Read the model definition and answer for the solid it produces. Units are mm, in the model's axes. A direction names the side the tool comes from. Coordinates: 2 decimals unless noted, no trailing zeros. Order: outer loops, then holes, each group sorted by start corner. A loop starts at its lowest first (then second) coordinate and runs counter-clockwise, first axis right, second up. Notation, with made-up numbers: (63.25, 60) -> (108.25, 60) arc R5 ccw to (108.25, 69) -> close; hole circle Ø6 at (-37.5, 23). An arc over 180 degrees is marked (long way). Answer in a Markdown table with one row per item.
from build123d import *

# Parameters (mm, degrees)
SKETCH1_W           = 73
SKETCH1_H           = 4
BOSS_EXTRUDE1_DEPTH = 200
SKETCH2_R           = 1.5
SKETCH2_W           = 40.5
SKETCH2_H           = 21
CUT_EXTRUDE1_DEPTH  = 2000


with BuildPart() as part:
    # Sketch1 → Boss-Extrude1 (new body)
    with BuildSketch(Plane(origin=(0, 0, 0), x_dir=(0, 0, -1), z_dir=(1, 0, 0))):
        Rectangle(SKETCH1_W, SKETCH1_H)
    extrude(amount=-BOSS_EXTRUDE1_DEPTH)

    # Sketch2 → Cut-Extrude1 (cut)
    with BuildSketch(Plane(origin=(0, 2, 0), x_dir=(1, 0, 0), z_dir=(0, 1, 0))):
        with Locations(Location((-186, 1.5, 0), (0, 0, 270))):
            Circle(SKETCH2_R)
        with Locations(Location((-133.5, 1.5, 0), (0, 0, 90))):
            Circle(SKETCH2_R)
        with Locations((-159.75, 1.5)):
            Rectangle(SKETCH2_W, SKETCH2_H)
    extrude(amount=-CUT_EXTRUDE1_DEPTH, mode=Mode.SUBTRACT)


solid = part.part
Q1. The part is cut by section A-A (x = -146). Write down the section's boundary in (y, z), then the cut area to 3 significant figures.
Outcome:
| item | result |
|---|---|
| outline | (-2, -36.5) -> (2, -36.5) -> (2, -12) -> (-2, -12) -> close; (-2, 9) -> (2, 9) -> (2, 36.5) -> (-2, 36.5) -> close |
| area | 208 mm² |
Q2. The part is cut by section B-B (y = -0.8). Write down the section's boundary in (x, z).
Outcome:
| item | result |
|---|---|
| outline | (-200, -36.5) -> (0, -36.5) -> (0, 36.5) -> (-200, 36.5) -> close; hole circle Ø3 at (-186, -1.5); hole (-180, -12) -> (-139.5, -12) -> (-139.5, 9) -> (-180, 9) -> close; hole circle Ø3 at (-133.5, -1.5) |
Q3. For faces 4 (the face through (-99, 0, -36.5)), 5 (the face through (-160, 0, -12)), determine the directions among +Z, -Z, +X, -X, +Y, -Y from which every point of the face is accessible in a straight line to the end or side of a thin tool.
Outcome:
| item | result |
|---|---|
| face 4 | -Z, +X, -X, +Y, -Y |
| face 5 | +Y, -Y |
Q4. For a pull along Z with two mould halves and no side action, classify faces 1 (the face through (-99, 0, 36.5)), 2 (the face through (-99, -2, 1)), 3 (the face through (-160, 0, 9)) as pulls with the +Z half, pulls with the -Z half, needs draft (parallel to the pull), parting line crosses it, or undercut.
Outcome:
| item | result |
|---|---|
| face 1 | pulls with the +Z half |
| face 2 | needs draft |
| face 3 | undercut |
Q5. Consider line 1 (X direction, y = 0.9, z = -1.5); line 2 (X direction, y = -0.35, z = 4.5); line 3 (Z direction, x = -169.5, y = -0.3). Determine where each line is inside the solid, lowest interval first.
Outcome:
| item | result |
|---|---|
| line 1 | -200 to -187.5, -184.5 to -180, -139.5 to -135, -132 to 0 |
| line 2 | -200 to -180, -139.5 to 0 |
| line 3 | -36.5 to -12, 9 to 36.5 |
Q6. Given pin 1 (4 mm diameter, centred on x = -186, z = -1.5, fed in from -Y), flat-ended and moving along its own axis, determine where the tip first touches the part or whether it passes through.
Outcome:
| item | result |
|---|---|
| pin 1 | y = -2 |
